from build123d import *

# Parameters (mm, degrees)
F1_DEPTH = 3.125
F2_W     = 5.9
F2_H     = 50.05
F2_W_2   = 50.05
F2_H_2   = 5.9
F3_DEPTH = 2
F4_R     = 2.6
F5_DEPTH = 25
F6_R     = 2
F8_DEPTH = 25
F9_R     = 3


# Not quite as in the source:
# - a feature names something its author has since deleted; it is built from what else it names


with BuildPart() as f1:
    # F0 (on Top) → F1 (new body)
    with BuildSketch(Plane.XY):
        with BuildLine():
            Line((35, 35), (15, 35))
            ThreePointArc((15, 35), (-4.5539513718, 4.5539513718), (-35, -15))
            Line((-35, -15), (-35, -35))
            Line((-35, -35), (35, -35))
            Line((35, -35), (35, 35))
        make_face()
    extrude(amount=F1_DEPTH)

    # F2 (on face) → F3 (join)
    with BuildSketch(Plane(origin=(0, 0, 0), x_dir=(1, 0, 0), z_dir=(0, 0, -1))):
        with Locations((25, -9.975)):
            Rectangle(F2_W, F2_H)
        with Locations((-9.975, 25)):
            Rectangle(F2_W_2, F2_H_2)
    extrude(amount=F3_DEPTH)

    # F4 (on face) → F5 (cut)
    with BuildSketch(Plane(origin=(0, 0, -2), x_dir=(1, 0, 0), z_dir=(0, 0, -1))):
        with Locations((25, -25)):
            Circle(F4_R)
        with Locations((25, 5)):
            Circle(F4_R)
        with Locations((5, 25)):
            Circle(F4_R)
        with Locations((-25, 25)):
            Circle(F4_R)
    extrude(amount=-F5_DEPTH, mode=Mode.SUBTRACT)

    # F6
    f6_edges = [f1.edges().sort_by_distance(p)[0] for p in [
        (35, 35, 1.5625),
        (15, 35, 1.5625),
        (-35, -15, 1.5625),
        (-35, -35, 1.5625),
        (35, -35, 1.5625),
    ]]
    fillet(f6_edges, radius=F6_R)

    # F7 (on Top) → F8 (cut)
    with BuildSketch(Plane.XY):
        with BuildLine():
            Line((15, -15), (15, 15))
            ThreePointArc((15, 15), (1.6961399442, -1.6961399442), (-15, -15))
            Line((-15, -15), (15, -15))
        make_face()
    extrude(amount=F8_DEPTH, mode=Mode.SUBTRACT)

    # F9
    f9_edges = [f1.edges().sort_by_distance(p)[0] for p in [
        (15, 15, 1.5625),
        (15, -15, 1.5625),
        (-15, -15, 1.5625),
    ]]
    fillet(f9_edges, radius=F9_R)


solid = f1.part
Here's how the part is built. I have some questions about the finished solid (model axes, mm). A direction names the side the tool comes from. Round coordinates to 2 decimals unless told otherwise and drop trailing zeros. Order: outer loops, then holes, each group sorted by start corner. A loop starts at its lowest first (then second) coordinate and runs counter-clockwise, first axis right, second up. Notation, with made-up numbers: M 50,55.25 L 66,55.25 A27 cw 66,71.25 Z; hole C -15.5,62 d7. An arc over 180 degrees is marked long. Return JSON: item names as keys, results as strings. Group by question number.
1. If we section it at C-C on z = -1.15: List the corners of the cut face in (x, y) for me.
2. If we mould it in two halves opening along Y, with no side actions, what happens to faces 5 (the face through (14.1, -14.14, 1.58)), 6 (the face through (-34.4, -34.43, 1.58)), 7 (the face through (-34.642, -15.236, 1.584))? For each: pulls with the +Y half, pulls with the -Y half, needs draft (parallel to the pull), parting line crosses it, or undercut.
3. If we section it at D-D on x = -4: List the corners of the cut face in (y, z) for me (3 decimals), then the cut area to 3 significant figures.
4. If we section it at B-B on x = 25: List the corners of the cut face in (y, z) for me (3 decimals), then the cut area to 3 significant figures.
5. Please list where these lines run through material, in increasing order: probe 1 along X at (y, z) = (-25, -0.65); probe 2 along X at (y, z) = (-25, 1.55); probe 3 along Y at (x, z) = (25, 0.95).
6. On a 3-axis mill with a long thin cutter (end or side, diameter ignored), from which of +Z, -Z, +X, -X, +Y, -Y can I reach the whole of each face in a straight line? I mean faces 1 (the face through (1.81, -1.58, 1.54)), 2 (the face through (25, -15.05, -1)), 3 (the face through (22.05, 10, -1)), 4 (the face through (15.05, -25, -1)). Say none if no direction works.
7. I'm going to push flat-ended pins straight in: pin 1 Ø10 at (x, y) = (2, -14) entering from +Z (3 decimals); pin 2 Ø1.5 at (x, y) = (20, -16.5) entering from -Z; pin 3 Ø1 at (y, z) = (15, -1) entering from +X; pin 4 Ø1.5 at (x, z) = (-20, -1) entering from -Y. Where does each tip first touch, or does it pass through?
8. If we section it at A-A on y = -25: List the corners of the cut face in (x, z) for me (3 decimals), then the cut area to 3 significant figures.
Reply:
{
 "1": {"outline": "M -35,-27.95 L 15.05,-27.95 L 15.05,-22.05 L -35,-22.05 Z; M 22.05,-15.05 L 27.95,-15.05 L 27.95,35 L 22.05,35 Z; hole C -25,-25 d5.2; hole C 5,-25 d5.2; hole C 25,-5 d5.2; hole C 25,25 d5.2"},
 "2": {"face 5": "undercut", "face 6": "pulls with the -Y half", "face 7": "pulls with the +Y half"},
 "3": {"outline": "M -35,0 L -27.95,0 L -27.95,-2 L -22.05,-2 L -22.05,0 L -15,0 L -15,3.125 L -35,3.125 Z; M -6.946,0 L 5.113,0 L 5.113,3.125 L -6.946,3.125 Z", "area": "112 mm^2"},
 "4": {"outline": "M -35,0 L -15.05,0 L -15.05,-2 L -7.6,-2 L -7.6,3.125 L -35,3.125 Z; M -2.4,-2 L 22.4,-2 L 22.4,3.125 L -2.4,3.125 Z; M 27.6,-2 L 35,-2 L 35,3.125 L 27.6,3.125 Z", "area": "266 mm^2"},
 "5": {"probe 1": "-35 to -27.6, -22.4 to 2.4, 7.6 to 15.05", "probe 2": "-35 to -27.6, -22.4 to 2.4, 7.6 to 35", "probe 3": "-35 to -7.6, -2.4 to 22.4, 27.6 to 35"},
 "6": {"face 1": "+Z, -Z", "face 2": "-Z, +X, -X, -Y", "face 3": "-Z, -X, +Y, -Y", "face 4": "-Z, +X, +Y, -Y"},
 "7": {"pin 1": "z = 3.125", "pin 2": "z = 0", "pin 3": "x = 27.95", "pin 4": "y = -27.95"},
 "8": {"outline": "M -35,-2 L -27.6,-2 L -27.6,3.125 L -35,3.125 Z; M -22.4,-2 L 2.4,-2 L 2.4,3.125 L -22.4,3.125 Z; M 7.6,-2 L 15.05,-2 L 15.05,0 L 35,0 L 35,3.125 L 7.6,3.125 Z", "area": "266 mm^2"}
}
